Drawing for the job (mm, zero at the part's lowest x, y, z). A direction names the side the tool comes from. Give positions to 0.01 mm unless a question says otherwise; leave off trailing zeros. Write each loop counter-clockwise with the first axis right and the second up, starting at its lowest first coordinate (ties: lowest second). Pieces come first, ordered by that corner, then holes. Notation, with made-up numbers: M -13,-26 L 29,-26 A9 cw 29,-18 Z; hole C 67,89 d7. An arc over 180 degrees is marked long. Use CSV: the item, a comma, the result in double quotes. Start each with the question number.
1. 3-axis set-ups, long thin cutter, end or side, ignore diameter. For the marked faces 1, 2 and 3: which of +Z, -Z, +X, -X, +Y, -Y reach the whole face in a straight line?
2. Band-saw the part on A-A, the plane x = 1.75. List the corners of the cut face in (y, z) (1 decimal).
3. Drop flat-ended pins along their axis: pin 1 Ø2.5 at (x, y) = (2.3, 2.3) entering from +Z; pin 2 Ø1 at (y, z) = (8.5, 0.5) entering from +X. Give the stop position or say it passes through.
4. Band-saw the part on D-D, the plane x = 4. List the corners of the cut face in (y, z), then the cut area to 3 significant figures.
5. Drill centre lines: line 1 along X through (y, z) = (5.75, 1.35); line 2 along X through (y, z) = (3, 1.45) (1 decimal); line 3 along Y through (x, z) = (1.5, 1.85) (1 decimal). Where is each one in solid material? Low to high. Write a range as from..to.
6. Mould opens along Y. For the marked faces 4, 5 and 6 say: pulls with the +Y half, pulls with the -Y half, needs draft (parallel to the pull), parting line crosses it, or undercut.
7. Band-saw the part on B-B, the plane y = 2.5. List the corners of the cut face in (x, z).
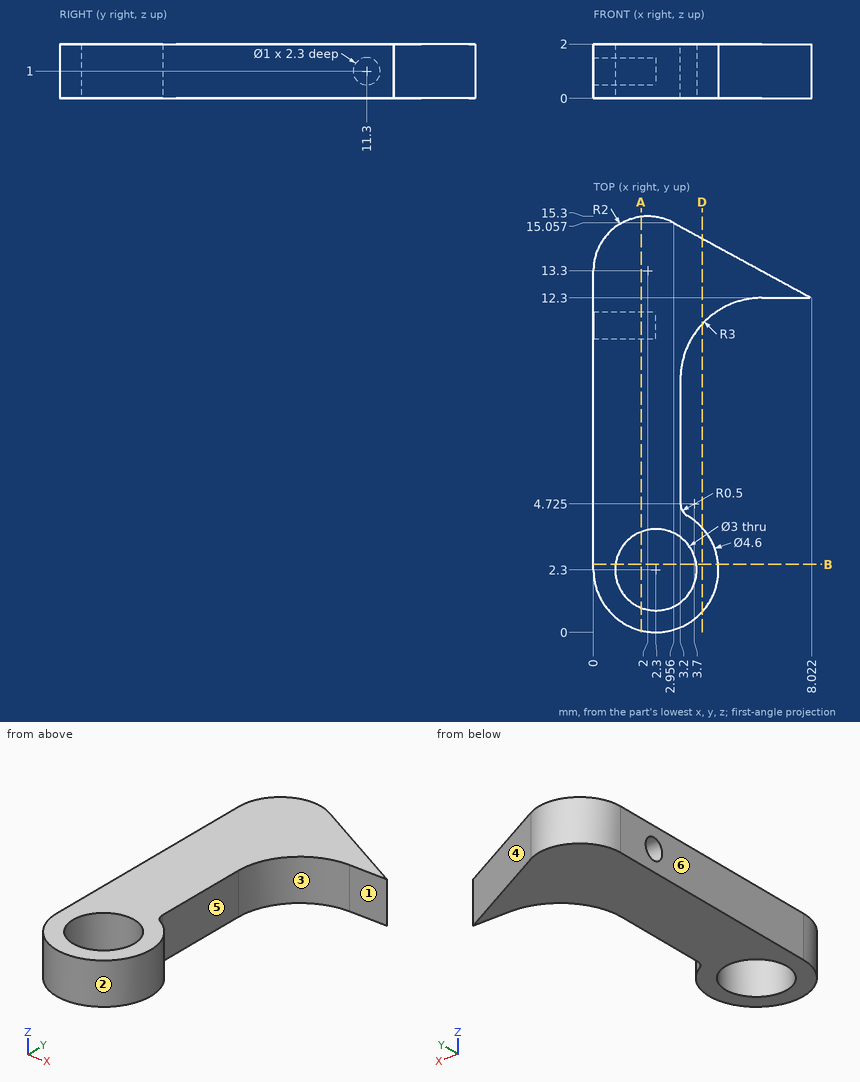
Output:
1,face 1,"+Z, -Z, +X, -Y"
1,face 2,"+Z, -Z"
1,face 3,"+Z, -Z, +X"
2,outline,"M 0.1,0 L 0.9,0 L 0.9,2 L 0.1,2 Z; M 3.7,0 L 15.3,0 L 15.3,2 L 3.7,2 Z; hole C 11.3,1 d1"
3,pin 1,"passes through"
3,pin 2,"stops at x = 3.2"
4,outline,"M 0.75,0 L 3.85,0 L 3.85,2 L 0.75,2 Z; M 11.34,0 L 14.49,0 L 14.49,2 L 11.34,2 Z"
4,area,"12.5 mm²"
5,line 1,"x = 0..3.2"
5,line 2,"x = 0..1, 3.6..4.5"
5,line 3,"y = 0.1..1, 3.6..15.2"
6,face 4,"pulls with the +Y half"
6,face 5,"undercut"
6,face 6,"needs draft"
7,outline,"M 0,0 L 0.81,0 L 0.81,2 L 0,2 Z; M 3.79,0 L 4.59,0 L 4.59,2 L 3.79,2 Z"
